```python
from build123d import *

# Parameters (mm, degrees)
EXTRUDE_1_DEPTH                    = 2.55
CUT_EXTRUDE_1_DEPTH                = 9.2
EXTRUDE_2_DEPTH                    = 3.8
SKETCH_4_W                         = 5.63
SKETCH_4_H                         = 1
CUT_EXTRUDE_2_DEPTH                = 3.8
CUT_EXTRUDE_3_REACH                = 16.939
CHAMFER_1_SIZE                     = 0.5
EXTRUDE_START                      = -3.6
SKETCH_6_W                         = 0.64
SKETCH_6_H                         = 0.64
EXTRUDE_3_DEPTH                    = 11.7
CHAMFER_2_SIZE                     = 0.2
PATTERN_LINEAR_1_COUNT             = 4
PATTERN_LINEAR_1_PITCH             = 2.54
CHAMFER_2_OF_PATTERN_LINEAR_1_SIZE = 0.2


with BuildPart() as part:
    # Эскиз1 → Бобышка-Вытянуть1 (new, symmetric)
    with BuildSketch(Plane(origin=(0, 0, 0), x_dir=(1, 0, 0), z_dir=(0, 1, 0))):
        Polygon((-4.955, -0.3), (4.955, -0.3), (4.955, 0), (5.655, 0), (5.655, -0.3), (6.355, -0.3), (6.355, -11.8), (-6.355, -11.8), (-6.355, -0.3), (-5.655, -0.3), (-5.655, 0), (-4.955, 0), align=None)
    extrude(amount=EXTRUDE_1_DEPTH, both=True)

    # Эскиз2 → Вырез-Вытянуть1 (cut)
    with BuildSketch(Plane.XY.offset(11.8)):
        Polygon((-5.355, 1.55), (-5.355, -1.55), (-3.14, -1.55), (-3.14, -2.55), (-1.94, -2.55), (-1.94, -1.55), (1.94, -1.55), (1.94, -2.55), (3.14, -2.55), (3.14, -1.55), (5.355, -1.55), (5.355, 1.55), (1.5, 1.55), (1.5, 2.55), (-1.5, 2.55), (-1.5, 1.55), align=None)
    extrude(amount=-CUT_EXTRUDE_1_DEPTH, mode=Mode.SUBTRACT)

    # Эскиз3 → Бобышка-Вытянуть2 (add)
    with BuildSketch(Plane.XY.offset(11.8)):
        Polygon((-3.815, 2.55), (-3.815, 4.05), (3.815, 4.05), (3.815, 2.55), (2.815, 2.55), (2.815, 3.05), (-2.815, 3.05), (-2.815, 2.55), align=None)
    extrude(amount=-EXTRUDE_2_DEPTH)

    # Эскиз4 → Вырез-Вытянуть2 (cut)
    with BuildSketch(Plane.XY.offset(11.8)):
        with Locations((0, 2.05)):
            Rectangle(SKETCH_4_W, SKETCH_4_H)
    extrude(amount=-CUT_EXTRUDE_2_DEPTH, mode=Mode.SUBTRACT)

    # Эскиз5 → Вырез-Вытянуть3 (cut, up to next)
    with BuildSketch(Plane(origin=(0, 4.05, 0), x_dir=(1, 0, 0), z_dir=(0, 1, 0)), mode=Mode.PRIVATE) as cut_extrude_3_sk1:
        with BuildLine():
            Line((2.815, -8), (2.815, -9.8))
            ThreePointArc((2.815, -9.8), (2.668553391, -10.153553391), (2.315, -10.3))
            Line((2.315, -10.3), (-2.315, -10.3))
            ThreePointArc((-2.315, -10.3), (-2.668553391, -10.153553391), (-2.815, -9.8))
            Line((-2.815, -9.8), (-2.815, -8))
            Line((-2.815, -8), (2.815, -8))
        make_face()
    cut_extrude_3_tool1 = extrude(cut_extrude_3_sk1.sketch, amount=-CUT_EXTRUDE_3_REACH, mode=Mode.PRIVATE) & part.part
    add(cut_extrude_3_tool1.solids().sort_by_distance((0, 4.05, 9.141324))[0], mode=Mode.SUBTRACT)

    # Фаска1
    chamfer_1_edges = [part.edges().sort_by_distance(p)[0] for p in [
        (2.1575, 1.55, 8),
        (-4.085, 1.55, 11.8),
        (-2.1575, 1.55, 8),
        (-5.355, 0, 11.8),
        (-4.2475, -1.55, 11.8),
        (0, -1.55, 11.8),
        (4.2475, -1.55, 11.8),
        (5.355, 0, 11.8),
        (4.085, 1.55, 11.8),
        (-2.815, 2.3, 11.8),
        (0, 3.05, 11.8),
        (2.815, 2.3, 11.8),
    ]]
    chamfer(chamfer_1_edges, length=CHAMFER_1_SIZE)

    # Эскиз6 → Бобышка-Вытянуть3 (add)
    with BuildSketch(Plane.XY.offset(0.3).offset(EXTRUDE_START)):
        with Locations((3.81, 0)):
            Rectangle(SKETCH_6_W, SKETCH_6_H)
    extrude_3 = extrude(amount=EXTRUDE_3_DEPTH)

    # Фаска2
    chamfer_2_edges = [part.edges().sort_by_distance(p)[0] for p in [
        (3.81, 0.32, 8.4),
        (4.13, 0, 8.4),
        (3.81, -0.32, 8.4),
        (3.49, 0, 8.4),
        (3.49, 0, -3.3),
        (3.81, 0.32, -3.3),
        (4.13, 0, -3.3),
        (3.81, -0.32, -3.3),
    ]]
    chamfer(chamfer_2_edges, length=CHAMFER_2_SIZE)

    # Линейный массив1: Бобышка-Вытянуть3 ×4
    with Locations(*[(-i * PATTERN_LINEAR_1_PITCH, 0, 0) for i in range(1, PATTERN_LINEAR_1_COUNT)]):
        add(extrude_3)

    # Фаска2 of Линейный массив1
    chamfer_2_of_pattern_linear_1_edges = [part.edges().sort_by_distance(p)[0] for p in [
        (1.27, 0.32, 8.4),
        (1.59, 0, 8.4),
        (1.27, -0.32, 8.4),
        (0.95, 0, 8.4),
        (0.95, 0, -3.3),
        (1.27, 0.32, -3.3),
        (1.59, 0, -3.3),
        (1.27, -0.32, -3.3),
        (-1.27, 0.32, 8.4),
        (-0.95, 0, 8.4),
        (-1.27, -0.32, 8.4),
        (-1.59, 0, 8.4),
        (-1.59, 0, -3.3),
        (-1.27, 0.32, -3.3),
        (-0.95, 0, -3.3),
        (-1.27, -0.32, -3.3),
        (-3.81, 0.32, 8.4),
        (-3.49, 0, 8.4),
        (-3.81, -0.32, 8.4),
        (-4.13, 0, 8.4),
        (-4.13, 0, -3.3),
        (-3.81, 0.32, -3.3),
        (-3.49, 0, -3.3),
        (-3.81, -0.32, -3.3),
    ]]
    chamfer(chamfer_2_of_pattern_linear_1_edges, length=CHAMFER_2_OF_PATTERN_LINEAR_1_SIZE)


solid = part.part
```
Input: part model. Units: mm. Frame: model coordinates. A direction names the side the tool comes from. Coordinates: 2 decimals unless noted, no trailing zeros. Write each loop counter-clockwise with the first axis right and the second up, starting at its lowest first coordinate (ties: lowest second). Pieces come first, ordered by that corner, then holes.
1) Material intervals for line 1 along X through (y, z) = (-1.75, 10.5) (3 decimals); line 2 along Y through (x, z) = (-3.75, 4.75); line 3 along Y through (x, z) = (1.25, 4.75), sorted ascending.
2) Section A-A on y = 2.75. Output: boundary loops of the cut face in (x, z) (3 decimals), and give its area (3 significant figures).
3) Mould query, pull axis X, two halves, no side actions, for faces 4 (the flat face through (0, -1.55, 7)), 5 (the flat face through (3, 3, 8)), 6 (the flat face through (-1.94, -2, 7)), 7 (the flat face through (3.815, 3, 10)). Classes: pulls with the +X half, pulls with the -X half, needs draft (parallel to the pull), parting line crosses it, or undercut.
4) Set-up query: faces 1 (the flat face through (-2.815, 3, 9)), 2 (the flat face through (-4, -1.55, 7)), 3 (the flat face through (0, 3.6, 10.3)). Return all of +Z, -Z, +X, -X, +Y, -Y with unobstructed straight access to the full face (end or side cutting, diameter ignored); none if empty.
5) Section C-C on z = -2. Output: boundary loops of the cut face in (x, y).
6) Pin query (flat end, axial travel): pin 1 Ø0.8 at (x, y) = (3, 3.5) entering from -Z; pin 2 Ø2 at (x, z) = (2, 0.5) entering from +Y; pin 3 Ø5 at (x, z) = (-3, 6.5) entering from +Y; pin 4 Ø1.5 at (x, y) = (4, -1) entering from +Z. Return the tip coordinate at first contact, or that it passes through.
7) Section B-B on x = 0.75. Output: boundary loops of the cut face in (y, z), and give its area (3 significant figures).
8) Section D-D on z = 9.5. Output: boundary loops of the cut face in (x, y) (3 decimals), and give its area (3 significant figures).
Check result:
1. line 1: x = -6.355 to -3.14, -1.94 to 1.94, 3.14 to 6.355
1. line 2: y = -2.55 to -1.55, -0.32 to 0.32, 1.55 to 2.55
1. line 3: y = -2.55 to -1.55, -0.32 to 0.32
2. outline: (-3.815, 8) - (-2.815, 8) - (-2.815, 11.3) - (-3.315, 11.8) - (-3.815, 11.8) - close; (2.815, 8) - (3.815, 8) - (3.815, 11.8) - (3.315, 11.8) - (2.815, 11.3) - close
2. area: 7.35 mm2
3. face 4: undercut
3. face 5: needs draft
3. face 6: undercut
3. face 7: pulls with the +X half
4. face 1: -Y
4. face 2: +Z
4. face 3: -Z, +Y
5. outline: (-4.13, -0.32) - (-3.49, -0.32) - (-3.49, 0.32) - (-4.13, 0.32) - close; (-1.59, -0.32) - (-0.95, -0.32) - (-0.95, 0.32) - (-1.59, 0.32) - close; (0.95, -0.32) - (1.59, -0.32) - (1.59, 0.32) - (0.95, 0.32) - close; (3.49, -0.32) - (4.13, -0.32) - (4.13, 0.32) - (3.49, 0.32) - close
6. pin 1: stops at z = 8
6. pin 2: stops at y = 2.55
6. pin 3: stops at y = 4.05
6. pin 4: stops at z = 11.5
7. outline: (-2.55, 0.3) - (2.55, 0.3) - (2.55, 2.6) - (-1.55, 2.6) - (-1.55, 11.3) - (-2.05, 11.8) - (-2.55, 11.8) - close; (3.05, 10.3) - (4.05, 10.3) - (4.05, 11.8) - (3.55, 11.8) - (3.05, 11.3) - close
7. area: 22.2 mm2
8. outline: (-6.355, -2.55) - (-3.14, -2.55) - (-3.14, -1.55) - (-5.355, -1.55) - (-5.355, 1.55) - (-2.815, 1.55) - (-2.815, 4.05) - (-3.815, 4.05) - (-3.815, 2.55) - (-6.355, 2.55) - close; (-1.94, -2.55) - (1.94, -2.55) - (1.94, -1.55) - (-1.94, -1.55) - close; (2.815, 1.55) - (5.355, 1.55) - (5.355, -1.55) - (3.14, -1.55) - (3.14, -2.55) - (6.355, -2.55) - (6.355, 2.55) - (3.815, 2.55) - (3.815, 4.05) - (2.815, 4.05) - close
8. area: 26.6 mm2
